For this review, use the dimensioned drawing (mm, ordinates from the lowest corner) and the shaded views. Give positions to 0.01 mm unless a question says otherwise; leave off trailing zeros. Order: outer loops, then holes, each group sorted by start corner. A loop starts at its lowest first (then second) coordinate and runs counter-clockwise, first axis right, second up. Notation, with made-up numbers: (47, 86) -> (105, 86) arc R20 ccw to (105, 111) -> close; hole circle Ø6 at (24.5, -6). An arc over 180 degrees is marked (long way). Return JSON: item names as keys, results as strings.
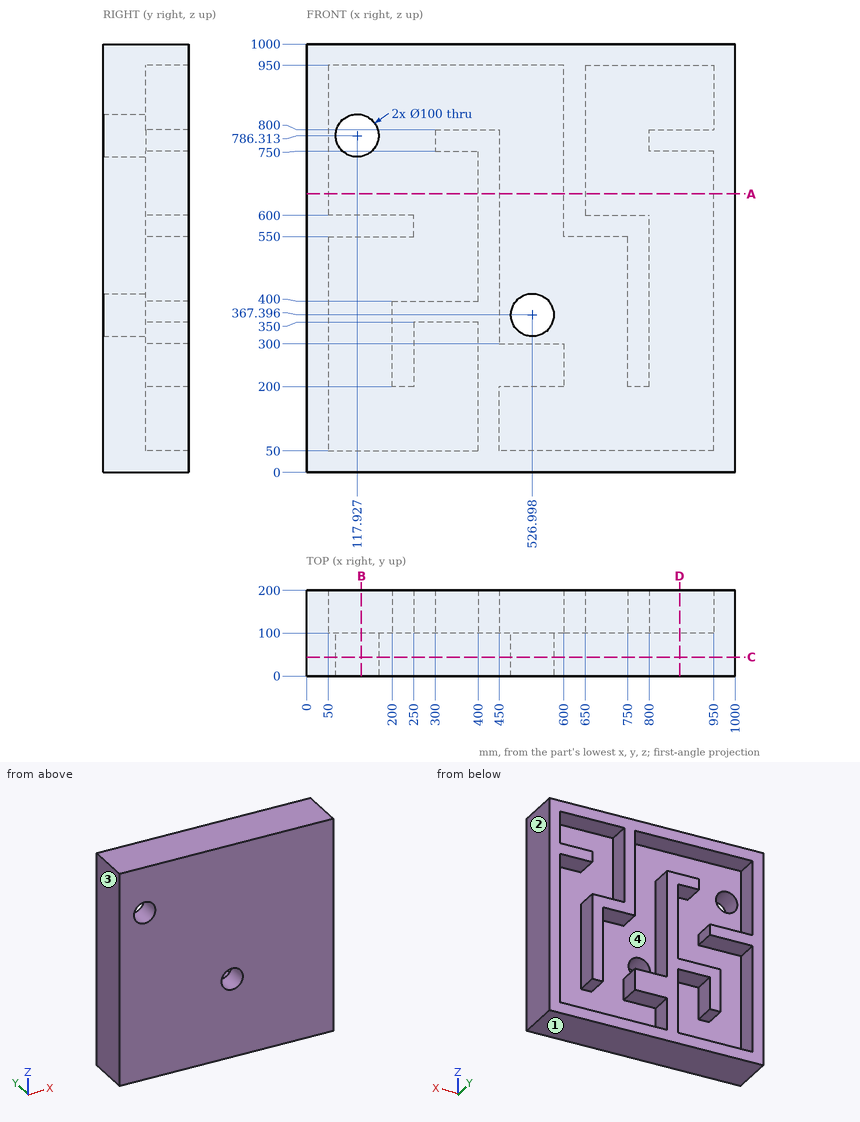
Item 1: Add section A-A (z = 650). Give the boundary of the cut face in (x, y).
Result set:
{"outline": "(0, 0) -> (1000, 0) -> (1000, 200) -> (950, 200) -> (950, 100) -> (650, 100) -> (650, 200) -> (600, 200) -> (600, 100) -> (450, 100) -> (450, 200) -> (400, 200) -> (400, 100) -> (50, 100) -> (50, 200) -> (0, 200) -> close"}
Item 2: Add section D-D (x = 870.5). Give the boundary of the cut face in (y, z), plus the area to 3 significant figures.
Result set:
{"outline": "(0, 0) -> (200, 0) -> (200, 50) -> (100, 50) -> (100, 750) -> (200, 750) -> (200, 800) -> (100, 800) -> (100, 950) -> (200, 950) -> (200, 1000) -> (0, 1000) -> close", "area": "115,000 mm^2"}
Item 3: Mouldability with a two-part tool opening along X and no side actions: class the marked faces 1, 2, 3 and 4 as released by +X, released by -X, zero draft, split by the parting line, or undercut.
Result set:
{"face 1": "zero draft", "face 2": "released by +X", "face 3": "released by -X", "face 4": "undercut"}
Item 4: Wall thickness on L1, parallel to X at y = 169, z = 71.5; L2, parallel to X at y = 152.5, z = 203.5; L3, parallel to Z at x = 896, y = 127.5: over which ranges is each line inside the solid? List them lowest first. Write a range as [from, to].
Result set:
{"L1": "x = [0, 50], [400, 450], [950, 1000]", "L2": "x = [0, 50], [200, 250], [400, 600], [750, 800], [950, 1000]", "L3": "z = [0, 50], [750, 800], [950, 1000]"}
Item 5: Add section B-B (x = 128). Give the boundary of the cut face in (y, z).
Result set:
{"outline": "(0, 0) -> (200, 0) -> (200, 50) -> (100, 50) -> (100, 550) -> (200, 550) -> (200, 600) -> (100, 600) -> (100, 737.34) -> (0, 737.34) -> close; (0, 835.29) -> (100, 835.29) -> (100, 950) -> (200, 950) -> (200, 1000) -> (0, 1000) -> close"}
Item 6: Add section C-C (y = 44). Give the boundary of the cut face in (x, z), plus the area to 3 significant figures.
Result set:
{"outline": "(0, 0) -> (1000, 0) -> (1000, 1000) -> (0, 1000) -> close; hole circle Ø100 at (117.93, 786.31); hole circle Ø100 at (527, 367.4)", "area": "984,000 mm^2"}
Item 7: For pin 1 (5 mm diameter, centred on x = 648, z = 185.5, fed in from +Y), flat-tipped, find the tip position at first contact; note if it passes through.
Result set:
{"pin 1": "stops at y = 100"}
